```python
from build123d import *

# Parameters (mm, degrees)
SCHIZZO1_R                   = 4
ESTRUSIONE_ESTRUSIONE1_DEPTH = 16
SMUSSO1_SIZE                 = 1
SCHIZZO6_R                   = 6.5
ESTRUSIONE_ESTRUSIONE3_DEPTH = 8
TAGLIO_ESTRUSIONE3_DEPTH     = 6
SCHIZZO8_R                   = 3.464101615
TAGLIO_ESTRUSIONE4_DEPTH     = 1
TAGLIO_ESTRUSIONE4_TAPER     = 45
RACCORDO1_R                  = 0.5
SCHIZZO9_R                   = 8
SCHIZZO9_R_2                 = 6.5
ESTRUSIONE_ESTRUSIONE4_DEPTH = 1
RACCORDO2_R                  = 0.1


with BuildPart() as part:
    # Schizzo1 → Estrusione-Estrusione1 (new body)
    with BuildSketch(Plane.XY):
        Circle(SCHIZZO1_R)
    extrude(amount=ESTRUSIONE_ESTRUSIONE1_DEPTH)

    # Smusso1
    smusso1_edges = [part.edges().sort_by_distance(p)[0] for p in [
        (-4, 0, 0),
    ]]
    chamfer(smusso1_edges, length=SMUSSO1_SIZE)

    # Schizzo6 → Estrusione-Estrusione3 (add)
    with BuildSketch(Plane.XY.offset(16)):
        Circle(SCHIZZO6_R)
    extrude(amount=ESTRUSIONE_ESTRUSIONE3_DEPTH)

    # Schizzo7 → Taglio-Estrusione3 (cut)
    with BuildSketch(Plane.XY.offset(24)):
        Polygon((1.732050808, 3), (-1.732050808, 3), (-3.464101615, 0), (-1.732050808, -3), (1.732050808, -3), (3.464101615, 0), align=None)
    extrude(amount=-TAGLIO_ESTRUSIONE3_DEPTH, mode=Mode.SUBTRACT)

    # Schizzo8 → Taglio-Estrusione4 (cut)
    with BuildSketch(Plane.XY.offset(24)):
        Circle(SCHIZZO8_R)
    extrude(amount=-TAGLIO_ESTRUSIONE4_DEPTH, taper=TAGLIO_ESTRUSIONE4_TAPER, mode=Mode.SUBTRACT)

    # Raccordo1
    raccordo1_edges = [part.edges().sort_by_distance(p)[0] for p in [
        (-6.5, 0, 24),
    ]]
    fillet(raccordo1_edges, radius=RACCORDO1_R)

    # Schizzo9 → Estrusione-Estrusione4 (add)
    with BuildSketch(Plane(origin=(0, 0, 16), x_dir=(-1, 0, 0), z_dir=(0, 0, -1))):
        Circle(SCHIZZO9_R)
        Circle(SCHIZZO9_R_2, mode=Mode.SUBTRACT)
    extrude(amount=-ESTRUSIONE_ESTRUSIONE4_DEPTH)

    # Raccordo2
    raccordo2_edges = [part.edges().sort_by_distance(p)[0] for p in [
        (-6.5, 0, 17),
        (8, 0, 17),
        (8, 0, 16),
    ]]
    fillet(raccordo2_edges, radius=RACCORDO2_R)


solid = part.part
```
The listing builds one solid part. Answer for the finished solid, in the listing's coordinates (mm). A direction names the side the tool comes from. Round coordinates to 2 decimals unless told otherwise and drop trailing zeros. Write each loop counter-clockwise with the first axis right and the second up, starting at its lowest first coordinate (ties: lowest second). Pieces come first, ordered by that corner, then holes. Notation, with made-up numbers: (-20.5, 8) -> (-14.5, 8) arc R27 cw to (-14.5, 25) -> close; hole circle Ø3 at (-34, 5.25). An arc over 180 degrees is marked (long way). Write item = value, one per line.
1) For a pull along X with two mould halves and no side action, classify faces 1 (the flat face through (0, 0, 0)), 2 (the cylindrical face through (-0.867, -3.905, 8.395)), 3 (the conical face through (2.808, 1.594, 23.765)) as released by +X, released by -X, zero draft, split by the parting line, or undercut.
Check values:
face_1 = zero draft
face_2 = split by the parting line
face_3 = undercut
2) Which of the six approach directions +Z, -Z, +X, -X, +Y, -Y give full straight-line access (tool end or side, diameter ignored) to faces 4 (the cylindrical face through (1.73, -7.81, 16.49)), 5 (the conical face through (-2.78, 1.63, 23.76))?
Check values:
face_4 = +Z, -Z
face_5 = +Z
3) Given pin 1 (6 mm diameter, centred on y = 2, z = 11.5, fed in from +X); pin 2 (1.7 mm diameter, centred on x = 0.5, z = 22, fed in from -Y); pin 3 (8 mm diameter, centred on x = 1.5, z = 5.5, fed in from -Y), each flat-ended and moving along its own axis, determine where each tip first touches the part or whether it passes through.
Check values:
pin_1 = 4
pin_2 = -6.5
pin_3 = -4
4) Section B-B on z = 4.75 is taken. Write down the section's boundary in (x, y).
Check values:
outline = circle Ø8 at (0, 0)
5) Section A-A on x = 0 is taken. Write down the section's boundary in (y, z), plus the area to 3 significant figures.
Check values:
outline = (-8, 16.1) arc R0.1 ccw to (-7.9, 16) -> (-4, 16) -> (-4, 1) -> (-3, 0) -> (3, 0) -> (4, 1) -> (4, 16) -> (7.9, 16) arc R0.1 ccw to (8, 16.1) -> (8, 16.9) arc R0.1 ccw to (7.9, 17) -> (6.6, 17) arc R0.1 cw to (6.5, 17.1) -> (6.5, 23.5) arc R0.5 ccw to (6, 24) -> (3.46, 24) -> (3, 23.54) -> (3, 18) -> (-3, 18) -> (-3, 23.54) -> (-3.46, 24) -> (-6, 24) arc R0.5 ccw to (-6.5, 23.5) -> (-6.5, 17.1) arc R0.1 cw to (-6.6, 17) -> (-7.9, 17) arc R0.1 ccw to (-8, 16.9) -> close
area = 198 mm²
6) Straight lines are drawn through the part: line 1 along Z through (x, y) = (-4.5, 2); line 2 along Z through (x, y) = (-3, -7); line 3 along X through (y, z) = (-2.5, 20). For each, find the intervals that lie inside material, in ascending order. Write a range as [from, to].
Check values:
line_1 = [16, 24]
line_2 = [16, 17]
line_3 = [-6, -2.02], [2.02, 6]
